Part print with two shaded views. Sizes in mm from the minimum x, y, z corner. Round coordinates to 2 decimals unless told otherwise and drop trailing zeros. Order: outer loops, then holes, each group sorted by start corner. A loop starts at its lowest first (then second) coordinate and runs counter-clockwise, first axis right, second up. Notation, with made-up numbers: (-2, 5) - (50, 5) arc R11 cw to (50, 18) - close; hole circle Ø4 at (47.25, 17.25). An arc over 180 degrees is marked (long way). Use one line per item in the form item = value.
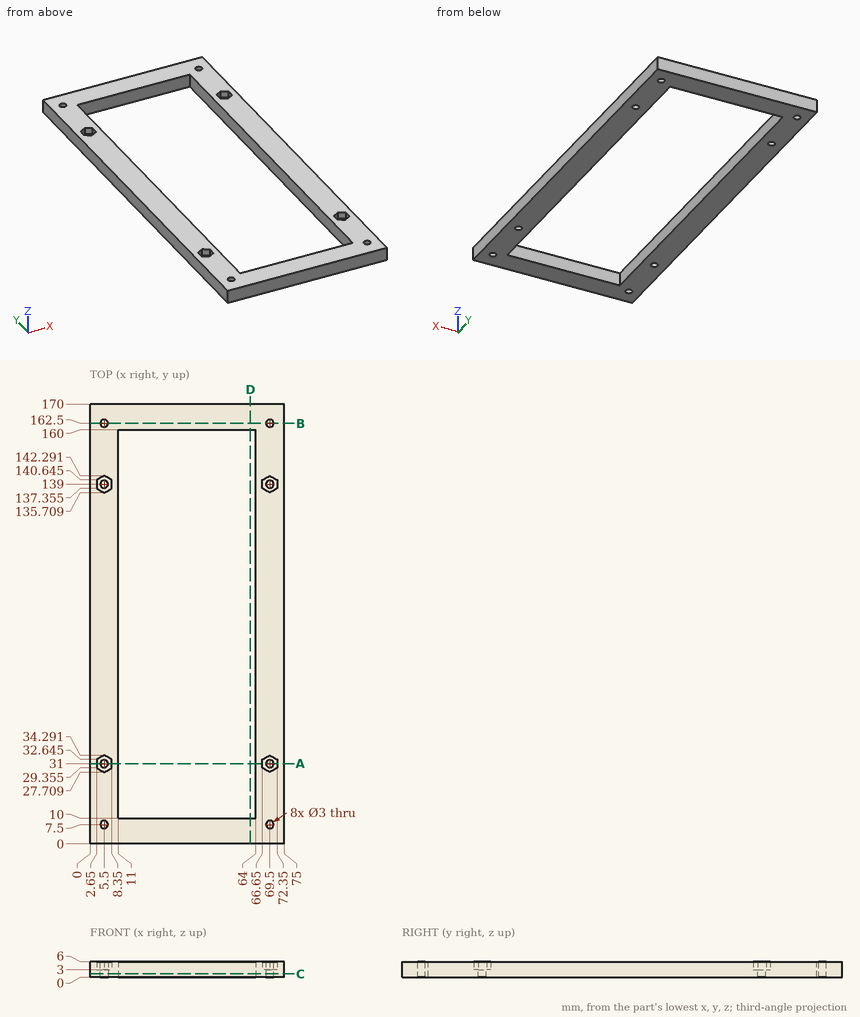
(1) Slice it at A-A on y = 31. Give the cut face in (x, z).
Report:
outline = (0, 0) - (4, 0) - (4, 3) - (2.65, 3) - (2.65, 6) - (0, 6) - close; (7, 0) - (11, 0) - (11, 6) - (8.35, 6) - (8.35, 3) - (7, 3) - close; (64, 0) - (68, 0) - (68, 3) - (66.65, 3) - (66.65, 6) - (64, 6) - close; (71, 0) - (75, 0) - (75, 6) - (72.35, 6) - (72.35, 3) - (71, 3) - close
(2) Pin check, flat tips, straight feed: pin 1 (2.5 mm diameter, centred on x = 69.5, y = 139, fed in from +Z); pin 2 (5 mm diameter, centred on x = 5.5, y = 139, fed in from +Z). Stop position of each tip, or through.
Report:
pin_1 = through
pin_2 = 3
(3) Probe probe 1 along Y at (x, z) = (5.5, 1.7); probe 2 along X at (y, z) = (7.5, 1.5); probe 3 along X at (y, z) = (114, 3.5). List the from-to ranges inside material, lowest first. Write a range as [from, to].
Report:
probe_1 = [0, 6], [9, 29.5], [32.5, 137.5], [140.5, 161], [164, 170]
probe_2 = [0, 4], [7, 68], [71, 75]
probe_3 = [0, 11], [64, 75]
(4) Slice it at C-C on z = 1.35. Count the separate pieces of the cut face and the enclosed holes in it, then the cut area to 3 significant figures.
Report:
separate_pieces = 1
enclosed_holes = 9
area = 4,740 mm2
(5) Slice it at B-B on y = 162.5. Give the cut face in (x, z), then the cut area to 3 significant figures.
Report:
outline = (0, 0) - (4, 0) - (4, 6) - (0, 6) - close; (7, 0) - (68, 0) - (68, 6) - (7, 6) - close; (71, 0) - (75, 0) - (75, 6) - (71, 6) - close
area = 414 mm2
(6) Slice it at D-D on x = 62. Give the cut face in (y, z), then the cut area to 3 significant figures.
Report:
outline = (0, 0) - (10, 0) - (10, 6) - (0, 6) - close; (160, 0) - (170, 0) - (170, 6) - (160, 6) - close
area = 120 mm2
